Verification items for the finished model (mm, model axes). Give positions to 0.01 mm unless a question says otherwise; leave off trailing zeros. Order: outer loops, then holes, each group sorted by start corner. A loop starts at its lowest first (then second) coordinate and runs counter-clockwise, first axis right, second up.
Autodesk Inventor part; units mm, degrees
ref_plane "YZ Plane" through (0, 0, 0) normal (1, 0, 0) x (0, 1, 0)
ref_plane "XZ Plane" through (0, 0, 0) normal (0, 1, 0) x (-1, 0, 0)
ref_plane "XY Plane" through (0, 0, 0) normal (0, 0, 1) x (1, 0, 0)
sketch "Sketch1" plane through (0, 0, 0) normal (0, 1, 0) x (-1, 0, 0)
  line L0 (71.1097, -38.0648) -> (71.1097, -13.0648)
  line L1 (71.1097, -13.0648) -> (74.1097, -13.0648)
  line L2 (74.1097, -13.0648) -> (74.1097, 11.9352)
  line L3 (74.1097, 11.9352) -> (71.1097, 11.9352)
  line L4 (71.1097, 11.9352) -> (71.1097, 36.9352)
  line L5 (-72.8903, -38.0648) -> (-72.8903, -13.0648)
  line L6 (-72.8903, 36.9352) -> (-72.8903, 11.9352)
  line L7 (-72.8903, -13.0648) -> (-75.8903, -13.0648)
  line L8 (-75.8903, -13.0648) -> (-75.8903, 11.9352)
  line L9 (-75.8903, 11.9352) -> (-72.8903, 11.9352)
  line L10 (71.1097, -38.0648) -> (-72.8903, -38.0648)
  line L11 (71.1097, 36.9352) -> (-72.8903, 36.9352)
  point P0 (0, 0)
extrude "Extrusion1" add sketch "Sketch1" along normal blind 3
sketch "Sketch2" plane through (0, 3, 0) normal (0, 1, 0) x (1, 0, 0)
  line L0 (-71.1097, -36.9352) -> (72.8903, -36.9352)
  line L1 (-66.1097, -31.9352) -> (-56.1097, -31.9352)
  line L2 (-56.1097, -31.9352) -> (-56.1097, -28.9352)
  line L3 (-56.1097, -28.9352) -> (-66.1097, -28.9352)
  line L4 (-66.1097, -28.9352) -> (-66.1097, -31.9352)
  line L5 (72.8903, 38.0648) -> (-71.1097, 38.0648)
  line L6 (-56.1097, 30.0648) -> (-66.1097, 30.0648)
  line L7 (-66.1097, 30.0648) -> (-66.1097, 33.0648)
  line L8 (-66.1097, 33.0648) -> (-56.1097, 33.0648)
  line L9 (-56.1097, 33.0648) -> (-56.1097, 30.0648)
  line L10 (67.8903, 33.0648) -> (57.8903, 33.0648)
  line L11 (57.8903, 33.0648) -> (57.8903, 30.0648)
  line L12 (57.8903, 30.0648) -> (67.8903, 30.0648)
  line L13 (67.8903, 30.0648) -> (67.8903, 33.0648)
  line L14 (67.8903, -31.9352) -> (57.8903, -31.9352)
  line L15 (57.8903, -31.9352) -> (57.8903, -28.9352)
  line L16 (57.8903, -28.9352) -> (67.8903, -28.9352)
  line L17 (67.8903, -28.9352) -> (67.8903, -31.9352)
  point P0 (0, 0)
extrude "Extrusion2" cut sketch "Sketch2" against normal blind 30
sketch "Sketch3" plane through (0, 3, 0) normal (0, 1, 0) x (1, 0, 0)
  line L0 (72.8903, 38.0648) -> (-71.1097, 38.0648)
  circle A0 centre (-14.1097, 28.0648) radius 5
  circle A1 centre (15.8903, 28.0648) radius 5
  line L1 (-71.1097, -36.9352) -> (72.8903, -36.9352)
  circle A2 centre (-14.1097, -26.9352) radius 5
  circle A3 centre (15.8903, -26.9352) radius 5
  point P0 (0, 0)
  dimension "d35" = 10
  dimension "d36" = 10
  dimension "d39" = 10
  dimension "d40" = 10
extrude "Extrusion3" cut sketch "Sketch3" against normal blind 30
sketch "Sketch4" plane through (0, 3, 0) normal (0, 1, 0) x (1, 0, 0)
  line L0 (-56.1097, 33.0648) -> (-56.1097, 30.0648)
  line L1 (-56.1097, 33.0648) -> (-41.1097, 33.0648)
  line L2 (-41.1097, 33.0648) -> (-41.1097, 30.0648)
  line L3 (-41.1097, 30.0648) -> (-56.1097, 30.0648)
  line L4 (-56.1097, 30.0648) -> (-56.1097, 33.0648)
  line L5 (57.8903, 33.0648) -> (42.8903, 33.0648)
  line L6 (42.8903, 33.0648) -> (42.8903, 30.0648)
  line L7 (42.8903, 30.0648) -> (57.8903, 30.0648)
  line L8 (57.8903, 30.0648) -> (57.8903, 33.0648)
  line L9 (-56.1097, -31.9352) -> (-66.1097, -31.9352)
  line L10 (-56.1097, -31.9352) -> (-41.1097, -31.9352)
  line L11 (-41.1097, -31.9352) -> (-41.1097, -28.9352)
  line L12 (-41.1097, -28.9352) -> (-56.1097, -28.9352)
  line L13 (-56.1097, -28.9352) -> (-56.1097, -31.9352)
  line L14 (57.8903, -31.9352) -> (57.8903, -28.9352)
  line L15 (57.8903, -31.9352) -> (42.8903, -31.9352)
  line L16 (42.8903, -31.9352) -> (42.8903, -28.9352)
  line L17 (42.8903, -28.9352) -> (57.8903, -28.9352)
  line L18 (57.8903, -28.9352) -> (57.8903, -31.9352)
  point P0 (0, 0)
  dimension "d43" = 15
  dimension "d44" = 15
extrude "Extrusion4" cut sketch "Sketch4" against normal blind 10
sketch "Sketch5" plane through (0, 3, 0) normal (0, 1, 0) x (1, 0, 0)
  circle A0 centre (-14.1097, 28.0648) radius 5
  circle A1 centre (-14.1097, 28.0648) radius 5
  circle A2 centre (15.8903, 28.0648) radius 5
  circle A3 centre (15.8903, 28.0648) radius 5
  circle A4 centre (15.8903, -26.9352) radius 5
  circle A5 centre (15.8903, -26.9352) radius 5
  circle A6 centre (-14.1097, -26.9352) radius 5
  circle A7 centre (-14.1097, -26.9352) radius 5
  point P0 (0, 0)
extrude "Extrusion5" add sketch "Sketch5" against normal blind 3
sketch "Sketch6" plane through (0, 3, 0) normal (0, 1, 0) x (1, 0, 0)
  line L0 (-74.1097, 13.0648) -> (-74.1097, -11.9352)
  line L1 (75.8903, -11.9352) -> (75.8903, 13.0648)
  line L2 (72.8903, 38.0648) -> (-71.1097, 38.0648)
  line L3 (0.8903, 38.0648) -> (0.8903, -36.9352)
  line L4 (-71.1097, -36.9352) -> (72.8903, -36.9352)
  circle A0 centre (-19.1097, 28.0648) radius 2
  circle A1 centre (20.8903, 28.0648) radius 2
  circle A2 centre (-19.1097, -26.9352) radius 2
  circle A3 centre (20.8903, -26.9352) radius 2
  point P0 (0, 0)
extrude "Extrusion6" cut sketch "Sketch6" against normal blind 3
properties part number "Level1 (Motoren)"
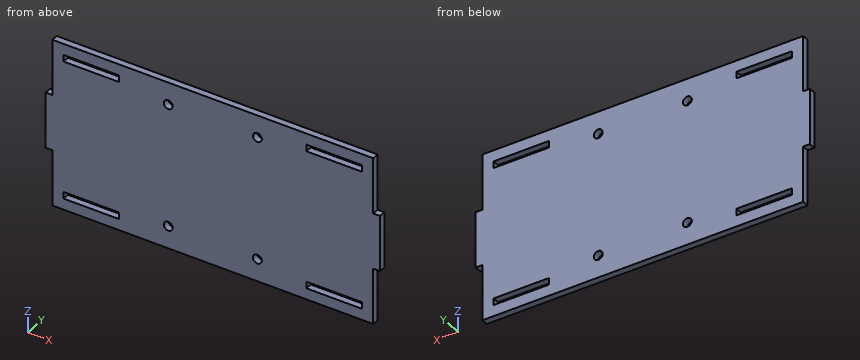
(1) Section check B-B, the plane y = 1.05. Give the number of separate pieces and of enclosed holes in the cut face, then the cut area to 3 significant figures.
Solved:
separate pieces: 1
enclosed holes: 8
area: 10,600 mm2
(2) Go/stop test with flat-tipped pins: pin 1 (1 mm diameter, centred on y = 0.5, z = -21, fed in from +X); pin 2 (0.9 mm diameter, centred on x = 74.5, y = 2, fed in from +Z); pin 3 (0.9 mm diameter, centred on y = 2, z = -31.5, fed in from -X). Record where each tip stops, or that it passes through.
Solved:
pin 1: stops at x = 72.89
pin 2: stops at z = 11.94
pin 3: stops at x = -71.11
(3) Section check C-C, the plane z = 19.5. Enter the section's corners in (x, y).
Solved:
outline: (-71.11, 0) - (72.89, 0) - (72.89, 3) - (-71.11, 3) - close
(4) Section check A-A, the plane x = -58. Enter the section's corners in (y, z), then the cut area to 3 significant figures.
Solved:
outline: (0, -38.06) - (3, -38.06) - (3, -33.06) - (0, -33.06) - close; (0, -30.06) - (3, -30.06) - (3, 28.94) - (0, 28.94) - close; (0, 31.94) - (3, 31.94) - (3, 36.94) - (0, 36.94) - close
area: 207 mm2
(5) Scan lines: line 1 (X direction, y = 1.45, z = 27); line 2 (Z direction, x = 64.5, y = 2.15); line 3 (X direction, y = 1.05, z = 30). Record each from-to range of solid material in increasing order.
Solved:
line 1: x = -71.11 to -21.11, -17.11 to 18.89, 22.89 to 72.89
line 2: z = -38.06 to -33.06, -30.06 to 28.94, 31.94 to 36.94
line 3: x = -71.11 to -66.11, -41.11 to 42.89, 67.89 to 72.89
